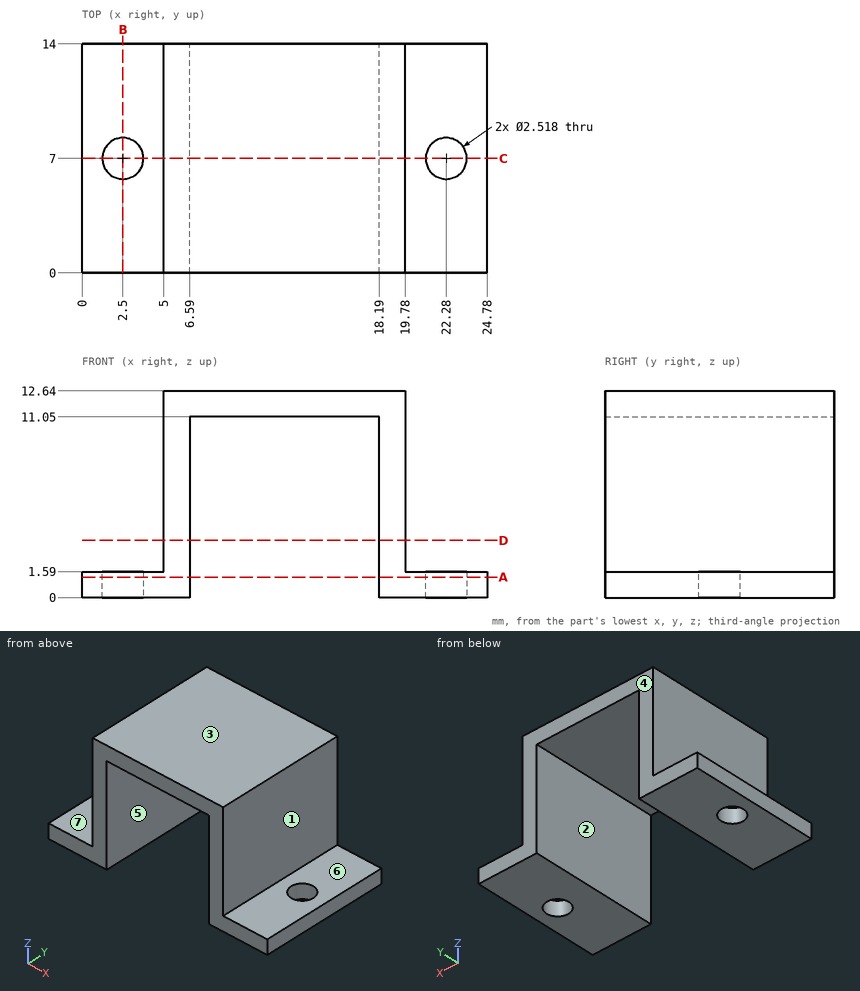
Part print with two shaded views. Sizes in mm from the minimum x, y, z corner. A direction names the side the tool comes from. Coordinates: 2 decimals unless noted, no trailing zeros. Write each loop counter-clockwise with the first axis right and the second up, starting at its lowest first coordinate (ties: lowest second). Pieces come first, ordered by that corner, then holes. Notation, with made-up numbers: M -20,-38 L 39,-38 A12 ccw 39,-29 Z; hole C 41.25,-17.5 d1. An arc over 180 degrees is marked long. Return JSON: item names as keys, results as strings.
Item 1: Slice it at C-C, the plane y = 7. Write the cut outline in (x, z).
Findings below:
{"outline": "M 0,0 L 1.24,0 L 1.24,1.59 L 0,1.59 Z; M 3.76,0 L 6.59,0 L 6.59,11.05 L 18.19,11.05 L 18.19,0 L 21.02,0 L 21.02,1.59 L 19.78,1.59 L 19.78,12.64 L 5,12.64 L 5,1.59 L 3.76,1.59 Z; M 23.54,0 L 24.78,0 L 24.78,1.59 L 23.54,1.59 Z"}
Item 2: Which spindle directions (+Z, -Z, +X, -X, +Y, -Y) get a long thin tool onto all of the face, cutting with end or side? Do the marked faces 4, 5, 6 and 7. Say none if no direction does.
Findings below:
{"face 4": "+Z, -Z, +X, -X, +Y", "face 5": "-Z, +Y, -Y", "face 6": "+Z, +X, +Y, -Y", "face 7": "+Z, -X, +Y, -Y"}
Item 3: Slice it at B-B, the plane x = 2.5. Write the cut outline in (y, z).
Findings below:
{"outline": "M 0,0 L 5.74,0 L 5.74,1.59 L 0,1.59 Z; M 8.26,0 L 14,0 L 14,1.59 L 8.26,1.59 Z"}
Item 4: Drop flat-ended pins along their axis: pin 1 Ø6 at (x, y) = (15, 5.5) entering from -Z; pin 2 Ø3 at (x, y) = (2.5, 7) entering from +Z; pin 3 Ø1.5 at (y, z) = (12, 5) entering from -X. Give the stop position or say it passes through.
Findings below:
{"pin 1": "stops at z = 11.05", "pin 2": "stops at z = 1.59", "pin 3": "stops at x = 5"}
Item 5: Two-plate mould, pull along X, no slides. Class the marked faces 1, 2 and 3: +X half, -X half, draft (parallel to the pull), parting line (faces both ways), or undercut.
Findings below:
{"face 1": "+X half", "face 2": "undercut", "face 3": "draft"}
Item 6: Slice it at D-D, the plane z = 3.5. Write the cut outline in (x, y), and give its area (3 significant figures).
Findings below:
{"outline": "M 5,0 L 6.59,0 L 6.59,14 L 5,14 Z; M 18.19,0 L 19.78,0 L 19.78,14 L 18.19,14 Z", "area": "44.5 mm2"}
Item 7: Probe line 1 (Y direction, x = 22.28, z = 0.85); line 2 (X direction, y = 9.5, z = 8.25); line 3 (Z direction, x = 21, y = 11.75). List the from-to ranges inside material, lowest first. Write a range as from..to.
Findings below:
{"line 1": "y = 0..5.74, 8.26..14", "line 2": "x = 5..6.59, 18.19..19.78", "line 3": "z = 0..1.59"}
Item 8: Slice it at A-A, the plane z = 1.25. Write the cut outline in (x, y), and give its area (3 significant figures).
Findings below:
{"outline": "M 0,0 L 6.59,0 L 6.59,14 L 0,14 Z; M 18.19,0 L 24.78,0 L 24.78,14 L 18.19,14 Z; hole C 2.5,7 d2.52; hole C 22.28,7 d2.52", "area": "175 mm2"}
